```python
from build123d import *

# Parameters (mm, degrees)
SKETCH1_R                = 17.5
BOSS_EXTRUDE1_DEPTH      = 50
SKETCH1_R_2              = 75
SKETCH1_R_3              = 72
BOSS_EXTRUDE1_2_DEPTH    = 50
SKETCH2_R                = 17.5
CUT_EXTRUDE1_DEPTH       = 10
BOSS_EXTRUDE2_DEPTH      = 2
CIRPATTERN1_COUNT        = 8
CUT_EXTRUDE2_START       = -8
SKETCH4_R                = 17.5
CUT_EXTRUDE2_DEPTH       = 8
SKETCH6_R                = 12.5
BOSS_EXTRUDE3_DEPTH      = 19
SKETCH7_R                = 3.5
CUT_EXTRUDE3_DEPTH       = 42
CUT_EXTRUDE4_DEPTH       = 3
CUT_EXTRUDE4_DEPTH_BACK  = 18
SKETCH8_R                = 2
BOSS_EXTRUDE4_DEPTH      = 51
BOSS_EXTRUDE4_DEPTH_BACK = 2
SKETCH9_R                = 79.710570968
SKETCH9_R_2              = 75


with BuildPart() as part:
    # Sketch1 → Boss-Extrude1 (new body)
    with BuildSketch(Plane(origin=(0, 0, 0), x_dir=(1, 0, 0), z_dir=(0, 1, 0))):
        with Locations(Location((0, 0, 0), (0, 0, 270))):
            Circle(SKETCH1_R)
    extrude(amount=BOSS_EXTRUDE1_DEPTH)

    # Sketch2 → Cut-Extrude1 (cut)
    with BuildSketch(Plane.XZ):
        with Locations(Location((0, 0, 0), (0, 0, 270))):
            Circle(SKETCH2_R)
    cut_extrude1 = extrude(amount=-CUT_EXTRUDE1_DEPTH, mode=Mode.SUBTRACT)

    # Mirror1: Cut-Extrude1 across plane
    add(cut_extrude1.mirror(Plane.ZX.offset(25)), mode=Mode.SUBTRACT)

    # Sketch4 → Cut-Extrude2 (cut)
    with BuildSketch(Plane(origin=(0, 40, 0), x_dir=(1, 0, 0), z_dir=(0, 1, 0)).offset(CUT_EXTRUDE2_START)):
        with Locations(Location((0, 0, 0), (0, 0, 90))):
            Circle(SKETCH4_R)
    extrude(amount=CUT_EXTRUDE2_DEPTH, mode=Mode.SUBTRACT)


with BuildPart() as body_2:
    # Sketch1 → Boss-Extrude1 2 (new body)
    with BuildSketch(Plane(origin=(0, 0, 0), x_dir=(1, 0, 0), z_dir=(0, 1, 0))):
        with Locations(Location((0, 0, 0), (0, 0, 270))):
            Circle(SKETCH1_R_2)
        with Locations(Location((0, 0, 0), (0, 0, 270))):
            Circle(SKETCH1_R_3, mode=Mode.SUBTRACT)
    extrude(amount=BOSS_EXTRUDE1_2_DEPTH)

    # Sketch3 → Boss-Extrude2 (add)
    with BuildSketch(Plane(origin=(0, 0, 0), x_dir=(0, 0, -1), z_dir=(1, 0, 0))):
        Polygon((16.718472528, 18.253836478), (16.718472528, 31.749663618), (73.745525638, 44.207029589), (73.745525638, 5.796470507), align=None)
    boss_extrude2 = extrude(amount=BOSS_EXTRUDE2_DEPTH)

    # CirPattern1: Boss-Extrude2 ×8 about axis
    cirpattern1_axis = Axis((0, 0, 0), (0, 1, 0))
    for i in range(1, CIRPATTERN1_COUNT):
        add(boss_extrude2.rotate(cirpattern1_axis, i * 360 / CIRPATTERN1_COUNT))


    add(part.part)  # Boss-Extrude3 merges part
    # Sketch6 → Boss-Extrude3 (add)
    with BuildSketch(Plane(origin=(0, 32, 0), x_dir=(1, 0, 0), z_dir=(0, 1, 0))):
        with Locations(Location((0, 0, 0), (0, 0, 270))):
            Circle(SKETCH6_R)
    extrude(amount=BOSS_EXTRUDE3_DEPTH)

    # Sketch7 → Cut-Extrude3 (cut)
    with BuildSketch(Plane(origin=(0, 51, 0), x_dir=(1, 0, 0), z_dir=(0, 1, 0))):
        with Locations(Location((0, 0, 0), (0, 0, 270))):
            Circle(SKETCH7_R)
    extrude(amount=-CUT_EXTRUDE3_DEPTH, mode=Mode.SUBTRACT)

    # Sketch8 → Cut-Extrude4 (cut, two sides: drawn at the far end of the back side and taken through both)
    with BuildSketch(Plane(origin=(0, 0, 0), x_dir=(0, 0, -1), z_dir=(1, 0, 0)).offset(-CUT_EXTRUDE4_DEPTH_BACK)):
        with Locations(Location((0, 41.737851991, 0), (0, 0, 180))):
            Circle(SKETCH8_R)
    extrude(amount=CUT_EXTRUDE4_DEPTH + CUT_EXTRUDE4_DEPTH_BACK, mode=Mode.SUBTRACT)

    # Sketch9 → Boss-Extrude4 (add, two sides: drawn at the far end of the back side and taken through both)
    with BuildSketch(Plane(origin=(0, 0, 0), x_dir=(1, 0, 0), z_dir=(0, 1, 0)).offset(-BOSS_EXTRUDE4_DEPTH_BACK)):
        with Locations(Location((0, 0, 0), (0, 0, 270))):
            Circle(SKETCH9_R)
        with Locations(Location((0, 0, 0), (0, 0, 270))):
            Circle(SKETCH9_R_2, mode=Mode.SUBTRACT)
    extrude(amount=BOSS_EXTRUDE4_DEPTH + BOSS_EXTRUDE4_DEPTH_BACK)


solid = body_2.part
```
Geometry: final body of the model. Coordinates: model frame, mm. A direction names the side the tool comes from. Round coordinates to 2 decimals unless told otherwise and drop trailing zeros. Write each loop counter-clockwise with the first axis right and the second up, starting at its lowest first coordinate (ties: lowest second). Pieces come first, ordered by that corner, then holes.
Item 1: Mould query, pull axis Z, two halves, no side actions, for faces 5 (the face through (51, 25, 2)), 6 (the face through (-3, 51, 3)). Classes: +Z half, -Z half, draft (parallel to the pull), parting line (faces both ways), or undercut.
Item 2: Section query D-D (x = -20.5). Return loops of the section in (y, z).
Item 3: Section query B-B (z = 45). Return loops of the section in (x, y), plus the area to 3 significant figures.
Item 4: Section query A-A (y = 30). Give the number of separate pieces and of enclosed holes in the cut face, plus the area to 3 significant figures.
Item 5: Set-up query: faces 1 (the face through (-47, -2, 59)), 2 (the face through (-51, 25, -2)), 3 (the face through (-30.635, 37.777, -32.029)), 4 (the face through (-32.57, 12.06, 31.18)). Return all of +Z, -Z, +X, -X, +Y, -Y with unobstructed straight access to the full face (end or side cutting, diameter ignored); none if empty.
Item 6: Section query C-C (x = 68). Return loops of the section in (y, z), plus the area to 3 significant figures.
Item 7: Material intervals for L1, parallel to Y at x = -8, z = 0; L2, parallel to Z at x = 55, y = 20; L3, parallel to Z at x = 15, y = 25.5, sorted ascending.
Item 8: Pin query (flat end, axial travel): P1, Ø19, axis at x = 57.5, y = 33.5, coming from the +Z side; P2, Ø6.5, axis at y = 41.74, z = 0, coming from the -X side; P3, Ø10, axis at x = 11.5, z = -6, coming from the -Y side; P4, Ø4, axis at x = -3.5, z = -42, coming from the +Y side. Return the tip coordinate at first contact, or that it passes through.
Completed:
1. face 5: undercut
1. face 6: draft
2. outline: (-2, -77.03) - (51, -77.03) - (51, -72.14) - (50, -72.14) - (50, -69.02) - (0, -69.02) - (0, -72.14) - (-2, -72.14) - close; (-2, 72.14) - (0, 72.14) - (0, 69.02) - (50, 69.02) - (50, 72.14) - (51, 72.14) - (51, 77.03) - (-2, 77.03) - close; (15.14, -23.33) - (34.87, -23.33) - (34.43, -20.5) - (15.57, -20.5) - close; (15.57, 20.5) - (16.01, 17.67) - (33.99, 17.67) - (34.43, 20.5) - close; (17.43, -2) - (32.58, -2) - (32.58, 0) - (17.43, 0) - close
3. outline: (-65.79, -2) - (-60, -2) - (-60, 0) - (-56.2, 0) - (-56.2, 50) - (-60, 50) - (-60, 51) - (-65.79, 51) - close; (-47.83, 7.57) - (-45, 8) - (-45, 42) - (-47.83, 42.44) - close; (-2, 12.08) - (0, 12.08) - (0, 37.93) - (-2, 37.93) - close; (42.17, 8.44) - (45, 8) - (45, 42) - (42.17, 41.56) - close; (56.2, 0) - (60, 0) - (60, -2) - (65.79, -2) - (65.79, 51) - (60, 51) - (60, 50) - (56.2, 50) - close
3. area: 1,240 mm2
4. separate pieces: 1
4. enclosed holes: 9
4. area: 5,470 mm2
5. face 1: +Z, -Z, +X, -X, -Y
5. face 2: +Y, -Y
5. face 3: +Y
5. face 4: -Y
6. outline: (-2, -41.59) - (51, -41.59) - (51, -31.64) - (50, -31.64) - (50, -23.66) - (0, -23.66) - (0, -31.64) - (-2, -31.64) - close; (-2, 31.64) - (0, 31.64) - (0, 23.66) - (50, 23.66) - (50, 31.64) - (51, 31.64) - (51, 41.59) - (-2, 41.59) - close; (7.05, 0) - (42.95, 0) - (42.95, 2) - (7.05, 2) - close
6. area: 1,920 mm2
7. L1: y = 10 to 39.74, 43.74 to 51
7. L2: z = -57.7 to -46.47, 0 to 2, 46.47 to 57.7
7. L3: z = -78.29 to -70.42, -15 to -12.17, -9.01 to 9.01, 15 to 17.83, 70.42 to 78.29
8. P1: stops at z = 63.64
8. P2: stops at x = -79.71
8. P3: stops at y = 10
8. P4: passes through
